Autodesk Inventor part; units mm, degrees
ref_plane "YZ Plane" through (0, 0, 0) normal (1, 0, 0) x (0, 1, 0)
ref_plane "XZ Plane" through (0, 0, 0) normal (0, 1, 0) x (-1, 0, 0)
ref_plane "XY Plane" through (0, 0, 0) normal (0, 0, 1) x (1, 0, 0)
sketch "Sketch1" plane through (0, 0, 0) normal (0, 1, 0) x (-1, 0, 0)
  circle A0 centre (11.3137, 0) radius 2.75
  circle A1 centre (0, 0) radius 15.739
  line L0 (0, -7.5575) -> (-6.545, -3.7788)
  line L1 (-6.545, -3.7788) -> (-6.545, 3.7788)
  line L2 (-6.545, 3.7788) -> (0, 7.5575)
  line L3 (0, 7.5575) -> (6.545, 3.7788)
  line L4 (6.545, 3.7788) -> (6.545, -3.7788)
  line L5 (6.545, -3.7788) -> (0, -7.5575)
  circle A2 centre (0, 11.3137) radius 2.75
  circle A3 centre (-11.3137, 0) radius 2.75
  circle A4 centre (0, -11.3137) radius 2.75
  circle A5 centre (0, 0) radius 3.4
  circle A6 centre (0, -11.3137) radius 4.4253
  circle A7 centre (11.3137, 0) radius 4.4253
  circle A8 centre (0, 11.3137) radius 4.4253
  circle A9 centre (-11.3137, 0) radius 4.4253
  line L6 (-2.8871, -5.8906) -> (-7.481, -13.8474)
  line L7 (-8.2517, -13.4024) -> (-3.6579, -5.4456)
  line L8 (-8.1837, -13.2847) -> (-7.413, -13.7297)
  point P0 (0, 0)
  dimension "d0" = 31.478
  dimension "d3" = 13.09
  dimension "d4" = 5.5
  dimension "d7" = 360
  dimension "d11" = 6.8
  dimension "d14" = 360
extrude "Extrusion1" add sketch "Sketch1" along normal blind 16.73 contours L7 L8 L6 A1 | A9 | A1 A8 L2 L1 L0 L7 | L6 L0 A6 A1 | L7 L0 L6 L8 | A7 | A6 L5 L4 L3 A8 A1 | A6 L0 L5 | A8 L3 L2 picked at (-1.3101, -7.6989) picked at (-1.3101, 7.6989)
extrude "Extrusion3" cut sketch "Sketch1" along normal blind 3 contours A0 | A9 | A7 | A6 L0 L5 | A8 L3 L2 | A6 L5 L0 | L2 L3 A8 | A2 | A3 | A4
extrude "Extrusion4" cut sketch "Sketch1" along normal blind 0.5 contours L7 L0 L6 L8
extrude "Extrusion5" cut sketch "Sketch1" along normal through all contours L7 L8 L6 A1
properties part number "GoBilda Mech Hub 0500 HexV2"
Source: CAD feature listing. Evaluate the final solid. Frame: model axes, mm. A direction names the side the tool comes from. Coordinates: 2 decimals unless noted, no trailing zeros. Write each loop counter-clockwise with the first axis right and the second up, starting at its lowest first coordinate (ties: lowest second). Pieces come first, ordered by that corner, then holes. Notation, with made-up numbers: M 72.25,72.25 L 95.25,72.25 A16 cw 95.25,88.25 Z; hole C 9.5,30.5 d8. An arc over 180 degrees is marked long. Answer as a JSON object with one key per item and string values.
1. Cut plane D-D on y = 12. State how many separate pieces and enclosed holes the cut face has, plus the area to 3 significant figures.
Evaluation:
{"separate pieces": "1", "enclosed holes": "5", "area": "535 mm^2"}
2. Cut plane A-A on z = -2. Output: boundary loops of the cut face in (x, y) (3 decimals).
Evaluation:
{"outline": "M -15.611,0 L -15.261,0 L -15.261,3 L -13.201,3 L -13.201,16.73 L -15.611,16.73 Z; M -9.426,3 L -7.366,3 L -7.366,0 L -6.545,0 L -6.545,16.73 L -9.426,16.73 Z; M 6.545,0 L 7.366,0 L 7.366,3 L 9.426,3 L 9.426,16.73 L 6.545,16.73 Z; M 13.201,3 L 15.261,3 L 15.261,0 L 15.611,0 L 15.611,16.73 L 13.201,16.73 Z"}
3. Cut plane B-B on x = 9. Output: boundary loops of the cut face in (y, z), plus the area to 3 significant figures.
Evaluation:
{"outline": "M 0,-12.91 L 16.73,-12.91 L 16.73,-1.49 L 3,-1.49 L 3,-3.77 L 0,-3.77 Z; M 0,3.77 L 3,3.77 L 3,1.49 L 16.73,1.49 L 16.73,12.91 L 0,12.91 Z", "area": "369 mm^2"}
4. Ray query, L1, parallel to X at y = 8.25, z = 0 (3 decimals); L2, parallel to Z at x = 2, y = 11.5; L3, parallel to X at y = 11, z = 2 (3 decimals). Return the intervals inside material, ascending.
Evaluation:
{"L1": "-15.739 to -14.064, -8.564 to -6.545, 6.545 to 8.564, 14.064 to 15.739", "L2": "-15.61 to -13.2, -9.43 to -6.4, 6.4 to 9.43, 13.2 to 15.61", "L3": "-15.611 to -13.201, -9.426 to -6.545, 6.545 to 9.426, 13.201 to 15.611"}
5. Draft query along Z for faces 1 (the flat face through (5, 0, -11)), 2 (the flat face through (6.545, 8, 0)). Return one class per face: released by +Z, released by -Z, zero draft, split by the parting line, or undercut.
Evaluation:
{"face 1": "zero draft", "face 2": "undercut"}
6. Contact query for flat-ended pins moving along their axis: P1, Ø7, axis at x = -11.31, z = 0, coming from the -Y side; P2, Ø5, axis at x = 10.5, y = 3, coming from the +Z side; P3, Ø4.5, axis at x = 0, z = -11.31, coming from the +Y side; P4, Ø3, axis at y = 7, z = 8.5, coming from the +X side. Output: stop coordinate, or through.
Evaluation:
{"P1": "y = 3", "P2": "z = 13.55", "P3": "through", "P4": "x = 14.1"}
7. Cut plane C-C on x = 1.5. Output: boundary loops of the cut face in (y, z).
Evaluation:
{"outline": "M 0,-15.67 L 16.73,-15.67 L 16.73,-13.62 L 3,-13.62 L 3,-15.48 L 0,-15.48 Z; M 0,-7.15 L 3,-7.15 L 3,-9.01 L 16.73,-9.01 L 16.73,-6.69 L 0,-6.69 Z; M 0,6.69 L 16.73,6.69 L 16.73,9.01 L 3,9.01 L 3,7.15 L 0,7.15 Z; M 0,15.48 L 3,15.48 L 3,13.62 L 16.73,13.62 L 16.73,15.67 L 0,15.67 Z"}
8. Access query for faces 3 (the flat face through (3.32, 8.25, 5.64)), 4 (the flat face through (-9, 3, -2)), 5 (the flat face through (-8, 0, 4)). Directions: +Z, -Z, +X, -X, +Y, -Y. A direction counts if a zero-diameter tool reaches every point of the face in a straight line with its end or side. Return the directions, or none.
Evaluation:
{"face 3": "+Y, -Y", "face 4": "-Y", "face 5": "+Z, -Z, +X, -X, -Y"}
